Input: part model. Units: mm. Frame: model coordinates. A direction names the side the tool comes from. Give positions to 0.01 mm unless a question says otherwise; leave off trailing zeros. Loops run counter-clockwise (first coordinate to the right, second up) from the corner with the lowest first, then second, coordinate; pieces in that order, holes last. Notation, with made-up numbers: (30.5, 78.25) -> (35.5, 78.25) arc R29 cw to (35.5, 109.25) -> close; hole circle Ø9 at (80, 85). An arc over 180 degrees is marked (long way). Answer as a JSON object with one key per item and string values. Group by question number.
```python
from build123d import *

# Parameters (mm, degrees)
ESQUISSE1_R         = 2.5
BOSS_EXTRU_1_DEPTH  = 3
CUT_EXTRUDE1_START  = -3
CUT_EXTRUDE1_DEPTH  = 3
BOSS_EXTRUDE1_DEPTH = 3
SKETCH1_R           = 2.75
CUT_EXTRUDE2_DEPTH  = 3


# Read off the part's stored shape, not the designer's step: Cut-Extrude1
with BuildPart() as part:
    # Esquisse1 → Boss.-Extru.1 (new body)
    with BuildSketch(Plane(origin=(0, 0, 0), x_dir=(1, 0, 0), z_dir=(0, 1, 0))):
        with BuildLine():
            Line((-85, 119.989574584), (153.28624341, 119.989574584))
            Line((153.28624341, 119.989574584), (153.28624341, -55.010425416))
            Line((153.28624341, -55.010425416), (-85, -55.010425416))
            ThreePointArc((-85, -55.010425416), (-92.071067812, -52.081493228), (-95, -45.010425416))
            Line((-95, -45.010425416), (-95, 109.989574584))
            ThreePointArc((-95, 109.989574584), (-92.071067812, 117.060642396), (-85, 119.989574584))
        make_face()
        with Locations(Location((141.78624341, -43.510425416, 0), (0, 0, 270))):
            Circle(ESQUISSE1_R, mode=Mode.SUBTRACT)
        with Locations(Location((141.78624341, 108.489574584, 0), (0, 0, 270))):
            Circle(ESQUISSE1_R, mode=Mode.SUBTRACT)
        with Locations(Location((-88.535533906, 113.52510849, 0), (0, 0, 270))):
            Circle(ESQUISSE1_R, mode=Mode.SUBTRACT)
        with Locations(Location((-88.535533906, -48.545959322, 0), (0, 0, 270))):
            Circle(ESQUISSE1_R, mode=Mode.SUBTRACT)
    extrude(amount=BOSS_EXTRU_1_DEPTH)

    # Cut-Extrude1 outline → Cut-Extrude1 (cut)
    with BuildSketch(Plane.XZ.offset(CUT_EXTRUDE1_START)):
        with BuildLine():
            Line((-26.534089411, -107.649444077), (41.026883272, -111.837107673))
            add(Edge.make_bspline(
                [(41.026883272, -111.837107673), (80.871896507, -115.445570806), (43.6868837, -98.824618367), (93.841601725, -105.501811245), (103.459361301, -42.407292201), (100.29035903, -19.379375914), (109.081082927, -3.387830236), (48.623008548, 72.204101039), (-7.977504863, 44.465677035)],
                knots=[0, 0, 0, 0, 0, 0, 0, 0, 0, 1, 1, 1, 1, 1, 1, 1, 1, 1], degree=8))
            Line((-7.977504863, 44.465677035), (-40.958080323, 28.587571847))
            add(Edge.make_bspline(
                [(-40.958080323, 28.587571847), (-63.284478038, 17.843514847), (-77.245184412, 4.644427122), (-85.775449686, -19.222136636), (-87.563403654, -31.078889142), (-86.988969289, -45.934210012), (-86.496578535, -48.869280426), (-84.771877477, -58.734159705), (-84.595340706, -59.308431064), (-82.980639435, -65.721995035), (-82.521559893, -67.446566753), (-82.039157422, -69.164892884)],
                knots=[0, 0, 0, 0, 1, 1, 1.52461883, 1.52461883, 1.947694096, 1.947694096, 2.583008028, 2.583008028, 2.817830116, 2.817830116, 2.817830116, 2.817830116], degree=3))
            add(Edge.make_bspline(
                [(-82.039157422, -69.164892884), (-78.230073131, -83.238962063), (-67.06916766, -105.136939227), (-26.534089411, -107.649444077)],
                knots=[0, 0, 0, 1, 1.688392895, 1.688392895, 1.688392895], degree=2))
        make_face()
    extrude(amount=CUT_EXTRUDE1_DEPTH, mode=Mode.SUBTRACT)

    # Sketch4 → Boss-Extrude1 (add)
    with BuildSketch(Plane(origin=(0, 0, 0), x_dir=(1, 0, 0), z_dir=(0, 1, 0))):
        with BuildLine():
            Line((93.302020541, 29.767829549), (97.480208944, 29.767829549))
            Line((97.480208944, 29.767829549), (95.391114743, 55.173684352))
            Line((95.391114743, 55.173684352), (91.102425061, 54.233284915))
            ThreePointArc((91.102425061, 54.233284915), (89.667608862, 49.644276713), (85.408121779, 47.41392616))
            ThreePointArc((85.408121779, 47.41392616), (79.969495118, 40.900759492), (86.482661786, 35.462132831))
            ThreePointArc((86.482661786, 35.462132831), (91.071669987, 34.027316631), (93.302020541, 29.767829549))
        make_face()
        with BuildLine():
            Line((36.624084675, 111.564206934), (36.331188094, 116.289605103))
            Line((36.331188094, 116.289605103), (21.485435183, 115.369413807))
            Line((21.485435183, 115.369413807), (21.384316793, 110.619593222))
            ThreePointArc((21.384316793, 110.619593222), (22.567491202, 110.213275552), (23.116811871, 109.089334924))
            ThreePointArc((23.116811871, 109.089334924), (29.47650759, 103.472016137), (35.093826377, 109.831711857))
            ThreePointArc((35.093826377, 109.831711857), (35.500144047, 111.014886266), (36.624084675, 111.564206934))
        make_face()
        with BuildLine():
            Line((-68.679115078, 99.310003258), (-77.197650928, 103.460523399))
            Line((-77.197650928, 103.460523399), (-90.092844695, 74.888102234))
            Line((-90.092844695, 74.888102234), (-81.269930428, 71.936494141))
            ThreePointArc((-81.269930428, 71.936494141), (-76.179120901, 76.650519158), (-69.246055906, 76.384092275))
            ThreePointArc((-69.246055906, 76.384092275), (-61.287768194, 79.327841024), (-64.231516944, 87.286128736))
            ThreePointArc((-64.231516944, 87.286128736), (-68.94554196, 92.376938263), (-68.679115078, 99.310003258))
        make_face()
        with BuildLine():
            Line((-86.523393512, 26.954917178), (-90.889130919, 29.767829549))
            Line((-90.889130919, 29.767829549), (-75.16950367, -12.427072891))
            Line((-75.16950367, -12.427072891), (-75.16950367, -2.91348489))
            ThreePointArc((-75.16950367, -2.91348489), (-74.944749705, 4.719117072), (-69.388760046, 9.957256624))
            ThreePointArc((-69.388760046, 9.957256624), (-65.912247557, 17.697661065), (-73.652651998, 21.174173554))
            ThreePointArc((-73.652651998, 21.174173554), (-81.28525396, 21.39892752), (-86.523393512, 26.954917178))
        make_face()
        with BuildLine():
            Line((8.366944085, -49.112206716), (11.747056213, -51.290065422))
            Line((11.747056213, -51.290065422), (-16.208470261, -45.189381197))
            Line((-16.208470261, -45.189381197), (-10.926193077, -43.04606622))
            ThreePointArc((-10.926193077, -43.04606622), (-7.791078178, -42.76925209), (-5.769954322, -40.356653937))
            ThreePointArc((-5.769954322, -40.356653937), (1.753445752, -36.432567887), (5.677531802, -43.955967961))
            ThreePointArc((5.677531802, -43.955967961), (5.954345932, -47.09108286), (8.366944085, -49.112206716))
        make_face()
    extrude(amount=BOSS_EXTRUDE1_DEPTH)

    # Sketch1 → Cut-Extrude2 (cut)
    with BuildSketch(Plane(origin=(0, 3, 0), x_dir=(1, 0, 0), z_dir=(0, 1, 0))):
        with Locations(Location((29.105319124, 109.46052339, 0), (0, 0, 270))):
            Circle(SKETCH1_R)
        with Locations(Location((85.945391782, 41.438029495, 0), (0, 0, 270))):
            Circle(SKETCH1_R)
        with Locations(Location((-0.04621126, -42.156310949, 0), (0, 0, 270))):
            Circle(SKETCH1_R)
        with Locations(Location((-66.738786425, 81.835110506, 0), (0, 0, 270))):
            Circle(SKETCH1_R)
        with Locations(Location((-71.520706022, 15.565715089, 0), (0, 0, 270))):
            Circle(SKETCH1_R)
    extrude(amount=-CUT_EXTRUDE2_DEPTH, mode=Mode.SUBTRACT)


solid = part.part
```
Q1. Section A-A on x = -23. Return the cut outline in (y, z), then the cut area to 3 significant figures.
Q2. Section B-B on y = 0.8. State how many separate pieces and enclosed holes the cut face has, then the cut area to 3 significant figures.
Q3. Pin query (flat end, axial travel): pin 1 Ø5 at (x, z) = (29.11, -109.46) entering from -Y. Return the tip coordinate at first contact, or that it passes through.
Q4. Set-up query: faces 4 (the face through (-68.91, 1.48, -92.28)), 5 (the face through (-91.99, 1.48, 52.16)). Return all of +Z, -Z, +X, -X, +Y, -Y with unobstructed straight access to the full face (end or side cutting, diameter ignored); none if empty.
Q5. Ray query, probe 1 along Z at (x, y) = (41, 0.7); probe 2 along Z at (x, y) = (22.5, 2.3); probe 3 along X at (y, z) = (2.7, -95). Return the intervals inside material, ascending.
Q6. Pull-direction query (Z, two-part tool) for faces 1 (the face through (-92.15, 1.48, -116.98)), 2 (the face through (110, 3, -34)), 3 (the face through (1.627, 1.479, 36.394)); classes: +Z half, -Z half, draft (parallel to the pull), parting line (faces both ways), or undercut.
Numbers:
{
 "1": {"outline": "(0, -119.99) -> (3, -119.99) -> (3, -107.87) -> (0, -107.87) -> close; (0, 37.23) -> (3, 37.23) -> (3, 55.01) -> (0, 55.01) -> close", "area": "89.7 mm²"},
 "2": {"separate pieces": "1", "enclosed holes": "10", "area": "20,700 mm²"},
 "3": {"pin 1": "passes through"},
 "4": {"face 4": "+Y, -Y", "face 5": "+Z, -X, +Y, -Y"},
 "5": {"probe 1": "z = -119.99 to -111.84, 43.04 to 55.01", "probe 2": "z = -119.99 to -110.27, 48.68 to 55.01", "probe 3": "x = -95 to -69.49, 73.12 to 153.29"},
 "6": {"face 1": "-Z half", "face 2": "draft", "face 3": "undercut"}
}
